```python
from build123d import *

# Parameters (mm, degrees)
SKETCH1_R           = 10
BOSS_EXTRUDE1_DEPTH = 6.35


with BuildPart() as part:
    # Sketch1 → Boss-Extrude1 (new body)
    with BuildSketch(Plane(origin=(0, 0, 0), x_dir=(1, 0, 0), z_dir=(0, 1, 0))):
        with BuildLine():
            ThreePointArc((29.929958333, 2.048803105), (24.270509831, 17.633557569), (11.19739331, 27.831966928))
            ThreePointArc((11.19739331, 27.831966928), (8.637024993, 26.58202963), (7.300338222, 29.098196883))
            ThreePointArc((7.300338222, 29.098196883), (-9.270509831, 28.531695489), (-23.009588682, 19.249904641))
            ThreePointArc((-23.009588682, 19.249904641), (-22.612024993, 16.428597802), (-25.418101183, 15.93487158))
            ThreePointArc((-25.418101183, 15.93487158), (-30, 0), (-25.418101183, -15.93487158))
            ThreePointArc((-25.418101183, -15.93487158), (-22.612024993, -16.428597802), (-23.009588682, -19.249904641))
            ThreePointArc((-23.009588682, -19.249904641), (-9.270509831, -28.531695489), (7.300338222, -29.098196883))
            ThreePointArc((7.300338222, -29.098196883), (8.637024993, -26.58202963), (11.19739331, -27.831966928))
            ThreePointArc((11.19739331, -27.831966928), (24.270509831, -17.633557569), (29.929958333, -2.048803105))
            ThreePointArc((29.929958333, -2.048803105), (27.95, 0), (29.929958333, 2.048803105))
        make_face()
        with Locations(Location((0, 0, 0), (0, 0, 270))):
            Circle(SKETCH1_R, mode=Mode.SUBTRACT)
    extrude(amount=BOSS_EXTRUDE1_DEPTH)


solid = part.part
```
Check sheet for the modelled part. Datum: model origin and axes. Units: mm. Round coordinates to 2 decimals unless told otherwise and drop trailing zeros. Loops run counter-clockwise (first coordinate to the right, second up) from the corner with the lowest first, then second, coordinate; pieces in that order, holes last. Notation, with made-up numbers: (-26.75, 86.5) -> (-11.75, 86.5) arc R27 ccw to (-11.75, 104.5) -> close; hole circle Ø10 at (-37, 54.5). An arc over 180 degrees is marked (long way). Write item = value, one per line. Start each with the question number.
1) Release check for a two-part mould opening along X. For faces 1 (the flat face through (13, 0, 0)), 2 (the cylindrical face through (-22.59, 3.13, -16.46)), 3 (the cylindrical face through (-30, 3, 0)), 4 (the cylindrical face through (-9.49, 3.13, 28.46)) record: released by +X, released by -X, zero draft, split by the parting line, or undercut.
2) Sectioned sample at B-B, the plane z = 0. Record the cut outline in (x, y), plus the area to 3 significant figures.
3) Sectioned sample at C-C, the plane y = 1. Record the cut outline in (x, z).
4) Sectioned sample at D-D, the plane z = 14.5. Record the cut outline in (x, y), plus the area to 3 significant figures.
5) Sectioned sample at A-A, the plane x = 0. Record the cut outline in (y, z).
6) Thickness scan on probe 1 along X at (y, z) = (4.75, 9); probe 2 along X at (y, z) = (2, 1.5); probe 3 along Z at (x, y) = (-8.5, 1.5). Record the ranges inside material, lowest first.
7) Gauge pin test, flat ends, axial feed: pin 1 Ø1 at (x, y) = (-2.5, 2) entering from -Z; pin 2 Ø12 at (x, z) = (0, 0) entering from -Y. Record the tip position at first contact, or that the pin passes through.
Results are:
q1.face_1 = zero draft
q1.face_2 = undercut
q1.face_3 = released by -X
q1.face_4 = split by the parting line
q2.outline = (-30, 0) -> (-10, 0) -> (-10, 6.35) -> (-30, 6.35) -> close; (10, 0) -> (27.95, 0) -> (27.95, 6.35) -> (10, 6.35) -> close
q2.area = 241 mm^2
q3.outline = (-25.42, -15.93) arc R2.05 cw to (-23.01, -19.25) arc R30 ccw to (7.3, -29.1) arc R2.05 cw to (11.2, -27.83) arc R30 ccw to (29.93, -2.05) arc R2.05 cw to (29.93, 2.05) arc R30 ccw to (11.2, 27.83) arc R2.05 cw to (7.3, 29.1) arc R30 ccw to (-23.01, 19.25) arc R2.05 cw to (-25.42, 15.93) arc R30 ccw to start; hole circle Ø20 at (0, 0)
q4.outline = (-26.26, 0) -> (26.26, 0) -> (26.26, 6.35) -> (-26.26, 6.35) -> close
q4.area = 334 mm^2
q5.outline = (0, -30) -> (6.35, -30) -> (6.35, -10) -> (0, -10) -> close; (0, 10) -> (6.35, 10) -> (6.35, 30) -> (0, 30) -> close
q6.probe_1 = -28.62 to -4.36, 4.36 to 28.62
q6.probe_2 = -29.96 to -9.89, 9.89 to 28.6
q6.probe_3 = -28.77 to -5.27, 5.27 to 28.77
q7.pin_1 = -29.93
q7.pin_2 = through
